Could you check a few things on this model? Use its own coordinates, in mm. Face numbers are marked on the shaded views. A direction names the side the tool comes from. Round coordinates to 2 decimals unless told otherwise and drop trailing zeros. Loops run counter-clockwise (first coordinate to the right, second up) from the corner with the lowest first, then second, coordinate; pieces in that order, holes last. Notation, with made-up numbers: (21.25, -23) -> (41.25, -23) arc R8 cw to (41.25, -9) -> close; hole circle Ø4 at (-37, 70.5). An arc over 180 degrees is marked (long way). Write each question's results on one line, items separated by ' | '.
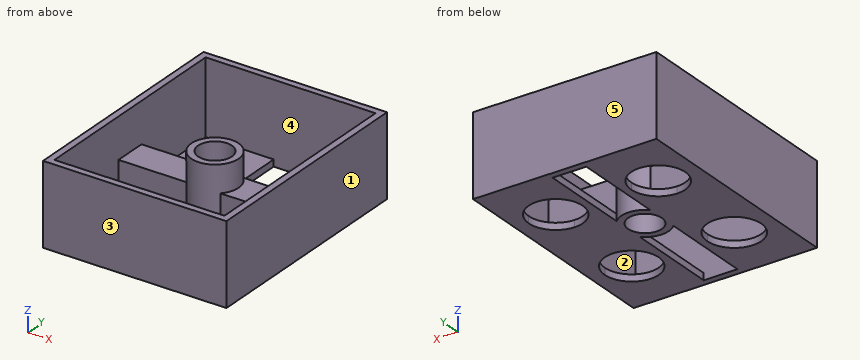
from build123d import *

# Parameters (mm, degrees)
F0_W     = 27.2
F0_H     = 34.2
F0_W_2   = 25.2
F0_H_2   = 32.2
F1_DEPTH = 12
F2_W     = 10.1
F2_H     = 32.2
F3_DEPTH = 1
F4_R     = 3.5
F4_R_2   = 2.5
F5_DEPTH = 10
F7_DEPTH = 25.4
F8_W     = 10.1
F8_H     = 4.89898
F9_DEPTH = 5


with BuildPart() as f1:
    # F0 (on Top) → F1 (new body)
    with BuildSketch(Plane.XY):
        Rectangle(F0_W, F0_H)
        Rectangle(F0_W_2, F0_H_2, mode=Mode.SUBTRACT)
    extrude(amount=F1_DEPTH)

    # F2 (on Top) → F3 (join)
    with BuildSketch(Plane.XY):
        with Locations((-7.55, 0)):
            Rectangle(F2_W, F2_H)
        with Locations((7.55, 0)):
            Rectangle(F2_W, F2_H)
    extrude(amount=F3_DEPTH)

    # F4 (on Top) → F5 (join)
    with BuildSketch(Plane.XY):
        Circle(F4_R)
        Circle(F4_R_2, mode=Mode.SUBTRACT)
    extrude(amount=F5_DEPTH)

    # F6 (on face) → F7 (cut)
    with BuildSketch(Plane.XY.offset(1)):
        with BuildLine():
            Line((-7.6, 4.1), (-7.6, 8.1))
            Line((-7.6, 8.1), (-3.6, 8.1))
            ThreePointArc((-3.6, 8.1), (-10.428427, 10.928427), (-7.6, 4.1))
        make_face()
        with BuildLine():
            ThreePointArc((11.6, 8.1), (7.6, 12.1), (3.6, 8.1))
            Line((3.6, 8.1), (7.6, 8.1))
            Line((7.6, 8.1), (7.6, 4.1))
            ThreePointArc((7.6, 4.1), (10.428427, 5.271573), (11.6, 8.1))
        make_face()
        with BuildLine():
            Line((7.6, 8.1), (3.6, 8.1))
            ThreePointArc((3.6, 8.1), (4.771573, 5.271573), (7.6, 4.1))
            Line((7.6, 4.1), (7.6, 8.1))
        make_face()
        with BuildLine():
            Line((-3.6, 8.1), (-7.6, 8.1))
            Line((-7.6, 8.1), (-7.6, 4.1))
            ThreePointArc((-7.6, 4.1), (-4.771573, 5.271573), (-3.6, 8.1))
        make_face()
        with BuildLine():
            Line((-7.6, -8.1), (-7.6, -4.1))
            ThreePointArc((-7.6, -4.1), (-10.428427, -10.928427), (-3.6, -8.1))
            Line((-3.6, -8.1), (-7.6, -8.1))
        make_face()
        with BuildLine():
            ThreePointArc((-3.6, -8.1), (-4.771573, -5.271573), (-7.6, -4.1))
            Line((-7.6, -4.1), (-7.6, -8.1))
            Line((-7.6, -8.1), (-3.6, -8.1))
        make_face()
        with BuildLine():
            ThreePointArc((11.6, -8.1), (10.428427, -5.271573), (7.6, -4.1))
            Line((7.6, -4.1), (7.6, -8.1))
            Line((7.6, -8.1), (3.6, -8.1))
            ThreePointArc((3.6, -8.1), (7.6, -12.1), (11.6, -8.1))
        make_face()
        with BuildLine():
            Line((7.6, -8.1), (7.6, -4.1))
            ThreePointArc((7.6, -4.1), (4.771573, -5.271573), (3.6, -8.1))
            Line((3.6, -8.1), (7.6, -8.1))
        make_face()
    extrude(amount=-F7_DEPTH, mode=Mode.SUBTRACT)

    # F8 (on face) → F9 (join)
    with BuildSketch(Plane.XY.offset(1)):
        with BuildLine():
            Line((-12.6, 2.44949), (-12.6, -2.44949))
            Line((-12.6, -2.44949), (-2.5, -2.44949))
            ThreePointArc((-2.5, -2.44949), (-3.5, 0), (-2.5, 2.44949))
            Line((-2.5, 2.44949), (-12.6, 2.44949))
        make_face()
        with Locations((7.55, 0)):
            Rectangle(F8_W, F8_H)
    extrude(amount=F9_DEPTH)


solid = f1.part
1) For the marked faces 1 and 2, which set-ups out of +Z, -Z, +X, -X, +Y, -Y let a thin tool reach every point of the face, with its end or its side?
Model answer:
face 1: +Z, -Z, +X, +Y, -Y | face 2: +Z
2) I want a section at B-B, the plane x = -10. Write out the boundary of the cut face in (y, z).
Model answer:
outline: (-17.1, 0) -> (-11.3, 0) -> (-11.3, 1) -> (-16.1, 1) -> (-16.1, 12) -> (-17.1, 12) -> close; (-4.9, 0) -> (4.9, 0) -> (4.9, 1) -> (2.45, 1) -> (2.45, 6) -> (-2.45, 6) -> (-2.45, 1) -> (-4.9, 1) -> close; (11.3, 0) -> (17.1, 0) -> (17.1, 12) -> (16.1, 12) -> (16.1, 1) -> (11.3, 1) -> close
3) I want a section at D-D, the plane y = -1.5. Write out the boundary of the cut face in (x, z).
Model answer:
outline: (-13.6, 0) -> (-2, 0) -> (-2, 10) -> (-3.16, 10) -> (-3.16, 6) -> (-12.6, 6) -> (-12.6, 12) -> (-13.6, 12) -> close; (2, 0) -> (13.6, 0) -> (13.6, 12) -> (12.6, 12) -> (12.6, 6) -> (3.16, 6) -> (3.16, 10) -> (2, 10) -> close
4) I want a section at C-C, the plane z = 11. Write out the boundary of the cut face in (x, y).
Model answer:
outline: (-13.6, -17.1) -> (13.6, -17.1) -> (13.6, 17.1) -> (-13.6, 17.1) -> close; hole (-12.6, -16.1) -> (12.6, -16.1) -> (12.6, 16.1) -> (-12.6, 16.1) -> close
5) I'm going to push flat-ended pins straight in: pin 1 (2 mm diameter, centred on x = 0.5, y = 1, fed in from +Z) (3 decimals); pin 2 (4 mm diameter, centred on x = 6, y = -1, fed in from +Z); pin 3 (5 mm diameter, centred on x = 9.5, y = 8, fed in from +Z). Where does each tip first touch, or does it pass through?
Model answer:
pin 1: passes through | pin 2: stops at z = 6 | pin 3: stops at z = 1
6) I want a section at A-A, the plane z = 6.5. Write out the boundary of the cut face in (x, y).
Model answer:
outline: (-13.6, -17.1) -> (13.6, -17.1) -> (13.6, 17.1) -> (-13.6, 17.1) -> close; circle Ø7 at (0, 0); hole (-12.6, -16.1) -> (12.6, -16.1) -> (12.6, 16.1) -> (-12.6, 16.1) -> close; hole circle Ø5 at (0, 0)
7) If we mould it in two halves opening along Y, with no side actions, what happens to the marked faces 3, 4 and 5? For each: released by +Y, released by -Y, zero draft, split by the parting line, or undercut.
Model answer:
face 3: released by -Y | face 4: undercut | face 5: released by +Y
8) I need wall thicknesses on line 1 (X direction, y = 8.1, z = 0.75); line 2 (Y direction, x = 5.5, z = 3.75); line 3 (Y direction, x = 0, z = 2). Which ranges of each line are inside material? Lowest first, please.
Model answer:
line 1: x = -13.6 to -11.6, -3.6 to -2.5, 2.5 to 3.6, 11.6 to 13.6 | line 2: y = -17.1 to -16.1, -2.45 to 2.45, 16.1 to 17.1 | line 3: y = -17.1 to -16.1, -3.5 to -2.5, 2.5 to 3.5, 16.1 to 17.1
